```python
from build123d import *

# Parameters (mm, degrees)
BOSS_EXTRUDE1_DEPTH    = 1.5
SKETCH2_W              = 41
SKETCH2_H              = 40
BOSS_EXTRUDE2_DEPTH    = 1.5
CONVERT_SOLID1_START   = -20
CONVERT_SOLID1_DEPTH   = 40
CONVERT_SOLID1_2_DEPTH = 40
M3_CLEARANCE_HOLE1_D   = 3.2
CIRPATTERN1_COUNT      = 6
SKETCH9_R              = 6.393167934
CUT_EXTRUDE1_DEPTH     = 54.525694764
M3_CLEARANCE_HOLE2_D   = 3.4
LPATTERN1_COUNT        = 2
LPATTERN1_PITCH        = 24
LPATTERN1_COPY_1_D     = 3.4
FILLET1_R              = 3
SKETCH12_R             = 10.195045523
CUT_EXTRUDE2_DEPTH     = 10


# Read off the part's stored shape, not the designer's step: Convert-Solid1
with BuildPart() as part:
    # Sketch1 → Boss-Extrude1 (new body)
    with BuildSketch(Plane(origin=(0, 0, 0), x_dir=(0, 0, -1), z_dir=(1, 0, 0))):
        with BuildLine():
            Line((-20, 0), (-20, -28))
            Line((-20, -28), (20, -28))
            Line((20, -28), (20, 0))
            ThreePointArc((20, 0), (0, 20), (-20, 0))
        make_face()
    extrude(amount=BOSS_EXTRUDE1_DEPTH)

    # Sketch2 → Boss-Extrude2 (add)
    with BuildSketch(Plane.XZ.offset(28)):
        with Locations((20.5, 0)):
            Rectangle(SKETCH2_W, SKETCH2_H)
    extrude(amount=-BOSS_EXTRUDE2_DEPTH)

    # Convert-Solid1 outline → Convert-Solid1 (cut)
    with BuildSketch(Plane.XY.offset(CONVERT_SOLID1_START)):
        with BuildLine():
            Line((0, -28), (2.262, -28))
            ThreePointArc((2.262, -28), (0.662524461, -27.337475539), (0, -25.738))
            Line((0, -25.738), (0, -28))
        make_face()
    extrude(amount=CONVERT_SOLID1_DEPTH, mode=Mode.SUBTRACT)

    # Convert-Solid1 2 outline → Convert-Solid1 2 (add)
    with BuildSketch(Plane.XY.offset(CONVERT_SOLID1_START)):
        with BuildLine():
            Line((1.5, -26.5), (2.262, -26.5))
            ThreePointArc((2.262, -26.5), (1.723184633, -26.276815367), (1.5, -25.738))
            Line((1.5, -25.738), (1.5, -26.5))
        make_face()
    extrude(amount=CONVERT_SOLID1_2_DEPTH)

    # M3 Clearance Hole1 (through all)
    with Locations(Plane.ZY):
        with Locations((-15.5, 0)):
            m3_clearance_hole1 = Hole(M3_CLEARANCE_HOLE1_D / 2)

    # CirPattern1: M3 Clearance Hole1 ×6 about axis
    cirpattern1_axis = Axis((0, 0, 0), (1, 0, 0))
    for i in range(1, CIRPATTERN1_COUNT):
        add(m3_clearance_hole1.rotate(cirpattern1_axis, i * 360 / CIRPATTERN1_COUNT), mode=Mode.SUBTRACT)

    # Sketch9 → Cut-Extrude1 (cut, through all)
    with BuildSketch(Plane.ZY):
        Circle(SKETCH9_R)
    extrude(amount=-CUT_EXTRUDE1_DEPTH, mode=Mode.SUBTRACT)

    # M3 Clearance Hole2 (through all)
    with Locations(Plane(origin=(0, -26.5, 0), x_dir=(1, 0, 0), z_dir=(0, 1, 0))):
        with Locations((33, 15)):
            m3_clearance_hole2 = Hole(M3_CLEARANCE_HOLE2_D / 2)

    # Mirror1: M3 Clearance Hole2 across plane
    add(m3_clearance_hole2.mirror(Plane.XY), mode=Mode.SUBTRACT)

    # LPattern1: M3 Clearance Hole2 ×2
    with Locations(*[(-i * LPATTERN1_PITCH, 0, 0) for i in range(1, LPATTERN1_COUNT)]):
        add(m3_clearance_hole2, mode=Mode.SUBTRACT)

    # LPattern1 copy 1 (through all)
    with Locations(Plane(origin=(-24, -26.5, 0), x_dir=(1, 0, 0), z_dir=(0, 1, 0))):
        with Locations((33, -15)):
            Hole(LPATTERN1_COPY_1_D / 2)

    # Fillet1
    fillet1_edges = [part.edges().sort_by_distance(p)[0] for p in [
        (41, -27.25, 20),
        (41, -27.25, -20),
    ]]
    fillet(fillet1_edges, radius=FILLET1_R)

    # Sketch12 → Cut-Extrude2 (cut)
    with BuildSketch(Plane(origin=(0, -26.5, 0), x_dir=(1, 0, 0), z_dir=(0, 1, 0))):
        with Locations(Location((20.131, 0, 0), (0, 0, 270))):
            Circle(SKETCH12_R)
    extrude(amount=-CUT_EXTRUDE2_DEPTH, mode=Mode.SUBTRACT)


solid = part.part
```
Here's how the part is built. I have some questions about the finished solid (model axes, mm). A direction names the side the tool comes from. Give positions to 0.01 mm unless a question says otherwise; leave off trailing zeros. Write each loop counter-clockwise with the first axis right and the second up, starting at its lowest first coordinate (ties: lowest second). Pieces come first, ordered by that corner, then holes. Notation, with made-up numbers: M -12.75,71.25 L 15.25,71.25 A25 ccw 15.25,89.25 Z; hole C -14,86.5 d1. An arc over 180 degrees is marked long. Put each result on its own line as item: value. Start each with the question number.
Item 1: If we section it at C-C, the plane z = -7: Write out the boundary of the cut face in (x, y) (3 decimals).
Item 2: If we section it at D-D, the plane y = 4: Write out the boundary of the cut face in (x, z), then the cut area to 3 significant figures.
Item 3: If we section it at A-A, the plane z = 0: Write out the boundary of the cut face in (x, y).
Item 4: Thinking about a two-plate mould opening in X: for faces 3 (the cylindrical face through (11.086, -27.24, 4.704)), 4 (the flat face through (1.5, -8, 0)), 5 (the cylindrical face through (10.7, -27.26, 14.93)), 6 (the flat face through (10, -27, 20)), which applies, +X half, -X half, draft (parallel to the pull), parting line (faces both ways), or undercut?
Item 5: I need wall thicknesses on L1, parallel to X at y = -27, z = -15; L2, parallel to Y at x = 16, z = 10; L3, parallel to Y at x = 0.4, z = -7.75. Which ranges of each line are inside material? Lowest first, please. Write a range as from..to.
Item 6: Will these pins go through, and if not, where does the flat tip stop? pin 1 (2.5 mm diameter, centred on y = 0, z = -15.5, fed in from +X); pin 2 (4.5 mm diameter, centred on x = 9, z = -15, fed in from -Y); pin 3 (4 mm diameter, centred on y = -13.42, z = 7.75, fed in from +X); pin 4 (1.5 mm diameter, centred on x = 20, z = 14, fed in from +Y).
Item 7: On a 3-axis mill with a long thin cutter (end or side, diameter ignored), from which of +Z, -Z, +X, -X, +Y, -Y can I reach the whole of each face in a straight line? I mean faces 1 (the flat face through (30, -26.5, -4)), 2 (the flat face through (30, -28, -4)). Say none if no direction works.
Item 8: If we section it at B-B, the plane x = 9: Write out the boundary of the cut face in (y, z).
Values:
1. outline: M 0,-25.738 A2.262 ccw 2.262,-28 L 12.719,-28 L 12.719,-26.5 L 2.262,-26.5 A0.762 cw 1.5,-25.738 L 1.5,-14.837 L 0,-14.837 Z; M 0,-12.01 L 1.5,-12.01 L 1.5,12.01 L 0,12.01 Z; M 0,14.837 L 1.5,14.837 L 1.5,18.735 L 0,18.735 Z; M 27.543,-28 L 41,-28 L 41,-26.5 L 27.543,-26.5 Z
2. outline: M 0,-19.6 L 1.5,-19.6 L 1.5,-4.99 L 0,-4.99 Z; M 0,4.99 L 1.5,4.99 L 1.5,19.6 L 0,19.6 Z
2. area: 43.8 mm²
3. outline: M 0,-25.74 A2.26 ccw 2.26,-28 L 9.94,-28 L 9.94,-26.5 L 2.26,-26.5 A0.76 cw 1.5,-25.74 L 1.5,-6.39 L 0,-6.39 Z; M 0,6.39 L 1.5,6.39 L 1.5,20 L 0,20 Z; M 30.33,-28 L 41,-28 L 41,-26.5 L 30.33,-26.5 Z
4. face 3: undercut
4. face 4: +X half
4. face 5: undercut
4. face 6: draft
5. L1: 0.38..7.3, 10.7..31.3, 34.7..41
5. L2: -28..-26.5
5. L3: -27.02..-15.02, -11.82..11.82, 15.02..18.44
6. pin 1: through
6. pin 2: y = -28
6. pin 3: x = 1.5
6. pin 4: y = -26.5
7. face 1: +Z, -Z, +X, +Y
7. face 2: +Z, -Z, +X, -X, -Y
8. outline: M -28,-20 L -26.5,-20 L -26.5,-16.7 L -28,-16.7 Z; M -28,-13.3 L -26.5,-13.3 L -26.5,13.3 L -28,13.3 Z; M -28,16.7 L -26.5,16.7 L -26.5,20 L -28,20 Z
